Can you work these out from the model? Positions are in its coordinate system, mm. A direction names the side the tool comes from. Give positions to 0.01 mm unless a question says otherwise; leave off trailing zeros. Order: outer loops, then holes, each group sorted by start corner. A loop starts at its lowest first (then second) coordinate and runs counter-clockwise, first axis right, second up. Notation, with made-up numbers: M 30,68 L 77,68 A33 ccw 77,97 Z; hole C -5.75,62.5 d10. An arc over 180 degrees is marked long. Answer as a JSON object with one key per item and string values.
```python
from build123d import *

# Parameters (mm, degrees)
SKETCH2_W           = 11
SKETCH2_H           = 2
SKETCH3_W           = 28.2
SKETCH3_H           = 29
BOSS_EXTRUDE1_DEPTH = 14.1
FILLET1_R           = 3
SKETCH5_W           = 15.5
SKETCH5_H           = 5.9
BOSS_EXTRUDE2_DEPTH = 2.5
SKETCH1_W           = 3
SKETCH1_H           = 147
CUT_EXTRUDE1_REACH  = 152.583
SKETCH7_R           = 1.5


with BuildPart() as part:
    # Sketch2 → Revolve2 (revolve)
    with BuildSketch(Plane(origin=(0, 0, 0), x_dir=(0, 0, -1), z_dir=(1, 0, 0)), mode=Mode.PRIVATE) as revolve2_sk:
        with Locations((-5.5, 1)):
            Rectangle(SKETCH2_W, SKETCH2_H)
    revolve(revolve2_sk.sketch.rotate(Axis((0, -54.281249734, 0), (0, 1, 0)), 180), axis=Axis((0, -54.281249734, 0), (0, 1, 0)))

    # Sketch3 → Boss-Extrude1 (add, symmetric)
    with BuildSketch(Plane(origin=(0, 0, 0), x_dir=(0, 0, -1), z_dir=(1, 0, 0))):
        with Locations((0, -14.5)):
            Rectangle(SKETCH3_W, SKETCH3_H)
    extrude(amount=BOSS_EXTRUDE1_DEPTH, both=True)

    # Fillet1
    fillet1_edges = [part.edges().sort_by_distance(p)[0] for p in [
        (-14.1, -14.5, -14.1),
        (14.1, -14.5, 14.1),
        (14.1, -14.5, -14.1),
        (-14.1, -14.5, 14.1),
    ]]
    fillet(fillet1_edges, radius=FILLET1_R)

    # Sketch5 → Boss-Extrude2 (add)
    with BuildSketch(Plane(origin=(14.1, 0, 0), x_dir=(0, 0, -1), z_dir=(1, 0, 0))):
        with Locations((0, -25.55)):
            Rectangle(SKETCH5_W, SKETCH5_H)
    extrude(amount=BOSS_EXTRUDE2_DEPTH)

    # Sketch1 → Revolve3 (revolve)
    with BuildSketch(Plane(origin=(0, 0, 0), x_dir=(0, 0, -1), z_dir=(1, 0, 0)), mode=Mode.PRIVATE) as revolve3_sk:
        with Locations((-1.5, 75.5)):
            Rectangle(SKETCH1_W, SKETCH1_H)
    revolve(revolve3_sk.sketch.rotate(Axis((0, -54.281249734, 0), (0, 1, 0)), 180), axis=Axis((0, -54.281249734, 0), (0, 1, 0)))

    # Sketch7 → Cut-Extrude1 (cut, up to next)
    with BuildSketch(Plane(origin=(0, 0, 0), x_dir=(1, 0, 0), z_dir=(0, 1, 0)), mode=Mode.PRIVATE) as cut_extrude1_sk1:
        with Locations(Location((-11.5, 11.5, 0), (0, 0, 270))):
            Circle(SKETCH7_R)
    cut_extrude1_tool1 = extrude(cut_extrude1_sk1.sketch, amount=-CUT_EXTRUDE1_REACH, mode=Mode.PRIVATE) & part.part
    # Sketch7 → Cut-Extrude1 (cut, up to next)
    with BuildSketch(Plane(origin=(0, 0, 0), x_dir=(1, 0, 0), z_dir=(0, 1, 0)), mode=Mode.PRIVATE) as cut_extrude1_sk2:
        with Locations(Location((-11.5, -11.5, 0), (0, 0, 270))):
            Circle(SKETCH7_R)
    cut_extrude1_tool2 = extrude(cut_extrude1_sk2.sketch, amount=-CUT_EXTRUDE1_REACH, mode=Mode.PRIVATE) & part.part
    # Sketch7 → Cut-Extrude1 (cut, up to next)
    with BuildSketch(Plane(origin=(0, 0, 0), x_dir=(1, 0, 0), z_dir=(0, 1, 0)), mode=Mode.PRIVATE) as cut_extrude1_sk3:
        with Locations(Location((11.5, -11.5, 0), (0, 0, 270))):
            Circle(SKETCH7_R)
    cut_extrude1_tool3 = extrude(cut_extrude1_sk3.sketch, amount=-CUT_EXTRUDE1_REACH, mode=Mode.PRIVATE) & part.part
    # Sketch7 → Cut-Extrude1 (cut, up to next)
    with BuildSketch(Plane(origin=(0, 0, 0), x_dir=(1, 0, 0), z_dir=(0, 1, 0)), mode=Mode.PRIVATE) as cut_extrude1_sk4:
        with Locations(Location((11.5, 11.5, 0), (0, 0, 270))):
            Circle(SKETCH7_R)
    cut_extrude1_tool4 = extrude(cut_extrude1_sk4.sketch, amount=-CUT_EXTRUDE1_REACH, mode=Mode.PRIVATE) & part.part
    add(cut_extrude1_tool1.solids().sort_by_distance((-11.5, 0, -11.5))[0], mode=Mode.SUBTRACT)
    add(cut_extrude1_tool2.solids().sort_by_distance((-11.5, 0, 11.5))[0], mode=Mode.SUBTRACT)
    add(cut_extrude1_tool3.solids().sort_by_distance((11.5, 0, 11.5))[0], mode=Mode.SUBTRACT)
    add(cut_extrude1_tool4.solids().sort_by_distance((11.5, 0, -11.5))[0], mode=Mode.SUBTRACT)


solid = part.part
```
1) For faces 1 (the face through (-0.9, 76.53, -2.86)), 2 (the face through (0, -29, 0)), which set-ups out of +Z, -Z, +X, -X, +Y, -Y let a thin tool reach every point of the face, with its end or its side?
Results found:
{"face 1": "+Y", "face 2": "+Z, -Z, +X, -X, -Y"}
2) I want a section at D-D on x = 7.5. Write out the boundary of the cut face in (y, z).
Results found:
{"outline": "M -29,-14.1 L 0,-14.1 L 0,-8.05 L 2,-8.05 L 2,8.05 L 0,8.05 L 0,14.1 L -29,14.1 Z"}
3) I want a section at B-B on x = 0. Write out the boundary of the cut face in (y, z), and give its area (3 significant figures).
Results found:
{"outline": "M -29,-14.1 L 0,-14.1 L 0,-11 L 2,-11 L 2,-3 L 149,-3 L 149,3 L 2,3 L 2,11 L 0,11 L 0,14.1 L -29,14.1 Z", "area": "1,740 mm²"}
4) Thinking about a two-plate mould opening in Z: for faces 3 (the face through (0, -15, 14.1)), 4 (the face through (0, 149, 0)), 5 (the face through (-12.4, -14.3, -12.7)), which applies, pulls with the +Z half, pulls with the -Z half, needs draft (parallel to the pull), parting line crosses it, or undercut?
Results found:
{"face 3": "pulls with the +Z half", "face 4": "needs draft", "face 5": "undercut"}
5) I'm going to push flat-ended pins straight in: pin 1 Ø5 at (x, y) = (2, 39.5) entering from -Z; pin 2 Ø8.5 at (x, z) = (-5.5, -5) entering from +Y; pin 3 Ø3 at (x, y) = (15, -25.5) entering from +Z. Where does each tip first touch, or does it pass through?
Results found:
{"pin 1": "stops at z = -3", "pin 2": "stops at y = 2", "pin 3": "stops at z = 12.9"}
6) I want a section at A-A on z = 0. Write out the boundary of the cut face in (x, y).
Results found:
{"outline": "M -14.1,-29 L 14.1,-29 L 14.1,-28.5 L 16.6,-28.5 L 16.6,-22.6 L 14.1,-22.6 L 14.1,0 L 11,0 L 11,2 L 3,2 L 3,149 L -3,149 L -3,2 L -11,2 L -11,0 L -14.1,0 Z"}
7) I want a section at C-C on y = 11.5. Write out the boundary of the cut face in (x, z), and give its area (3 significant figures).
Results found:
{"outline": "C 0,0 d6", "area": "28.3 mm²"}
8) I need wall thicknesses on L1, parallel to X at y = -20.25, z = -11.5; L2, parallel to Y at x = -12, z = -1.75; L3, parallel to Y at x = 4.5, z = 5.75. Which ranges of each line are inside material? Lowest first, please.
Results found:
{"L1": "x = -14.07 to -13, -10 to 10, 13 to 14.07", "L2": "y = -29 to 0", "L3": "y = -29 to 2"}
